Here's how the part is built. I have some questions about the finished solid (model axes, mm). A direction names the side the tool comes from. Give positions to 0.01 mm unless a question says otherwise; leave off trailing zeros. Loops run counter-clockwise (first coordinate to the right, second up) from the corner with the lowest first, then second, coordinate; pieces in that order, holes last. Notation, with made-up numbers: (-4.5, 45) - (21.5, 45) arc R23 ccw to (21.5, 61) - close; hole circle Ø6 at (88, 81.25). An arc over 180 degrees is marked (long way). Use one line per item in the form item = value.
from build123d import *

# Parameters (mm, degrees)
BOSS_EXTRUDE1_DEPTH   = 85
BOSS_EXTRUDE1_2_DEPTH = 85
SKETCH1_5_W           = 40
SKETCH1_5_H           = 89.12
SKETCH1_5_W_2         = 20
SKETCH1_5_H_2         = 20
BOSS_EXTRUDE2_DEPTH   = 40
SKETCH1_6_R           = 9
BOSS_EXTRUDE3_DEPTH   = 50
CUT_EXTRUDE1_DEPTH    = 43
CUT_EXTRUDE2_DEPTH    = 86
SKETCH4_W             = 30
SKETCH4_H             = 13.637460926
CUT_EXTRUDE3_DEPTH    = 103


with BuildPart() as part:
    # Sketch1 → Boss-Extrude1 (new body)
    with BuildSketch(Plane(origin=(0, 0, 0), x_dir=(1, 0, 0), z_dir=(0, 1, 0))):
        Polygon((-30, -44.56), (-20, -44.56), (-20, 44.56), (-30, 44.56), (-30, 18), (-30, -18), align=None)
    extrude(amount=BOSS_EXTRUDE1_DEPTH)



with BuildPart() as body_2:
    # Sketch1 → Boss-Extrude1 2 (new body)
    with BuildSketch(Plane(origin=(0, 0, 0), x_dir=(1, 0, 0), z_dir=(0, 1, 0))):
        Polygon((20, 44.56), (20, -44.56), (30, -44.56), (30, -18), (30, 18), (30, 44.56), align=None)
    extrude(amount=BOSS_EXTRUDE1_2_DEPTH)


with BuildPart() as part_1:
    add(part.part)

    add(body_2.part)  # Boss-Extrude2 merges body 2
    # Sketch1_5 → Boss-Extrude2 (add)
    with BuildSketch(Plane(origin=(0, 0, 0), x_dir=(1, 0, 0), z_dir=(0, 1, 0))):
        Rectangle(SKETCH1_5_W, SKETCH1_5_H)
        Rectangle(SKETCH1_5_W_2, SKETCH1_5_H_2, mode=Mode.SUBTRACT)
    extrude(amount=BOSS_EXTRUDE2_DEPTH)

    # Sketch1_6 → Boss-Extrude3 (add)
    with BuildSketch(Plane(origin=(0, 0, 0), x_dir=(1, 0, 0), z_dir=(0, 1, 0))):
        with BuildLine():
            Line((-48, -18), (-30, -18))
            Line((-30, -18), (-30, 18))
            Line((-30, 18), (-48, 18))
            ThreePointArc((-48, 18), (-66, 0), (-48, -18))
        make_face()
        with Locations((-48, 0)):
            Circle(SKETCH1_6_R, mode=Mode.SUBTRACT)
        with BuildLine():
            Line((30, 18), (30, -18))
            Line((30, -18), (48, -18))
            ThreePointArc((48, -18), (66, 0), (48, 18))
            Line((48, 18), (30, 18))
        make_face()
        with Locations((48, 0)):
            Circle(SKETCH1_6_R, mode=Mode.SUBTRACT)
    extrude(amount=BOSS_EXTRUDE3_DEPTH)

    # Sketch2 → Cut-Extrude1 (cut, symmetric)
    with BuildSketch(Plane(origin=(0, 0, 0), x_dir=(0, 0, -1), z_dir=(1, 0, 0))):
        with BuildLine():
            Line((-30.56, 67), (30.56, 67))
            ThreePointArc((30.56, 67), (34.56, 71), (30.56, 75))
            Line((30.56, 75), (-30.56, 75))
            ThreePointArc((-30.56, 75), (-34.56, 71), (-30.56, 67))
        make_face()
    extrude(amount=CUT_EXTRUDE1_DEPTH, both=True, mode=Mode.SUBTRACT)

    # Sketch3 → Cut-Extrude2 (cut)
    with BuildSketch(Plane(origin=(30, 0, 0), x_dir=(0, 0, -1), z_dir=(1, 0, 0))):
        with BuildLine():
            ThreePointArc((-44.56, 71), (-40.459494937, 80.899494937), (-30.56, 85))
            Line((-30.56, 85), (-44.56, 85))
            Line((-44.56, 85), (-44.56, 71))
        make_face()
        with BuildLine():
            Line((44.56, 85), (30.56, 85))
            ThreePointArc((30.56, 85), (40.459494937, 80.899494937), (44.56, 71))
            Line((44.56, 71), (44.56, 85))
        make_face()
    extrude(amount=-CUT_EXTRUDE2_DEPTH, mode=Mode.SUBTRACT)

    # Sketch4 → Cut-Extrude3 (cut)
    with BuildSketch(Plane.XY.offset(44.56)):
        with Locations((-0.820162859, 23.181269537)):
            Rectangle(SKETCH4_W, SKETCH4_H)
    extrude(amount=-CUT_EXTRUDE3_DEPTH, mode=Mode.SUBTRACT)


solid = part_1.part
(1) If we section it at D-D (z = -32.5): List the corners of the cut face in (x, y) for me.
Geometry says:
outline = (-30, 0) - (30, 0) - (30, 67.5) - (20, 67.5) - (20, 40) - (-20, 40) - (-20, 67.5) - (-30, 67.5) - close; (-30, 74.5) - (-20, 74.5) - (-20, 84.86) - (-30, 84.86) - close; (20, 74.5) - (30, 74.5) - (30, 84.86) - (20, 84.86) - close; hole (-15.82, 16.36) - (14.18, 16.36) - (14.18, 30) - (-15.82, 30) - close
(2) If I drill on probe 1 along X at (y, z) = (15, 0); probe 2 along X at (y, z) = (28.5, 0); probe 3 along X at (y, z) = (75.5, -11.5), over which ranges is the centre line in solid material (lowest first)?
Geometry says:
probe_1 = -66 to -57, -39 to -10, 10 to 39, 57 to 66
probe_2 = -66 to -57, -39 to -15.82, 14.18 to 39, 57 to 66
probe_3 = -30 to -20, 20 to 30
(3) If we section it at B-B (z = 14.5): List the corners of the cut face in (x, y) for me.
Geometry says:
outline = (-58.67, 0) - (58.67, 0) - (58.67, 50) - (30, 50) - (30, 67) - (20, 67) - (20, 40) - (-20, 40) - (-20, 67) - (-30, 67) - (-30, 50) - (-58.67, 50) - close; (-30, 75) - (-20, 75) - (-20, 85) - (-30, 85) - close; (20, 75) - (30, 75) - (30, 85) - (20, 85) - close; hole (-15.82, 16.36) - (14.18, 16.36) - (14.18, 30) - (-15.82, 30) - close
(4) Thinking about a two-plate mould opening in Y: for faces 1 (the flat face through (-39, 25, 18)), 2 (the flat face through (0, 40, -11)), 3 (the cylindrical face through (25.07, 71.09, 34.56)), 4 (the flat face through (-25, 67, 0)), which applies, pulls with the +Y half, pulls with the -Y half, needs draft (parallel to the pull), parting line crosses it, or undercut?
Geometry says:
face_1 = needs draft
face_2 = pulls with the +Y half
face_3 = undercut
face_4 = undercut
(5) For faces 5 (the cylindrical face through (-24.93, 70.91, -34.56)), 6 (the flat face through (-20, 62, 1)), 7 (the flat face through (-36, 50, 0)), 8 (the flat face through (0, 8, -10)), which set-ups out of +Z, -Z, +X, -X, +Y, -Y let a thin tool reach every point of the face, with its end or its side?
Geometry says:
face_5 = +X, -X
face_6 = +Z, -Z, +Y
face_7 = +Z, -Z, -X, +Y
face_8 = +Y, -Y
(6) If we section it at A-A (y = 63.5): List the corners of the cut face in (x, z) for me, plus the area to 3 significant figures.
Geometry says:
outline = (-30, -44.56) - (-20, -44.56) - (-20, 44.56) - (-30, 44.56) - close; (20, -44.56) - (30, -44.56) - (30, 44.56) - (20, 44.56) - close
area = 1,780 mm²
(7) For P1, Ø11, axis at y = 36.5, z = -0.5, coming from the -X side; P2, Ø8, axis at x = 0, y = 19, coming from the -Z side; P3, Ø8, axis at y = 66, z = 6.5, coming from the +X side; P4, Ø15, axis at x = -6.5, z = -20, coming from the +Y side, each with a flat end and sliding along its axis, tell me the tip position at first contact or that it passes through.
Geometry says:
P1 = -66
P2 = -44.56
P3 = 30
P4 = 40
(8) If we section it at C-C (x = 42.5): List the corners of the cut face in (y, z) for me, plus the area to 3 significant figures.
Geometry says:
outline = (0, -18) - (50, -18) - (50, -7.12) - (0, -7.12) - close; (0, 7.12) - (50, 7.12) - (50, 18) - (0, 18) - close
area = 1,090 mm²
